Input: part model. Units: mm. Frame: model coordinates. Face numbers are marked on the shaded views. A direction names the side the tool comes from. Give positions to 0.01 mm unless a question says otherwise; leave off trailing zeros. Write each loop counter-clockwise with the first axis right and the second up, starting at its lowest first coordinate (ties: lowest second). Pieces come first, ordered by that corner, then holes. Notation, with made-up numbers: (-17, 36.5) - (12, 36.5) arc R30 cw to (12, 71.5) - close; hole circle Ø9 at (36.25, 26.25). An arc over 180 degrees is marked (long way). Answer as CSV lines item,"result".
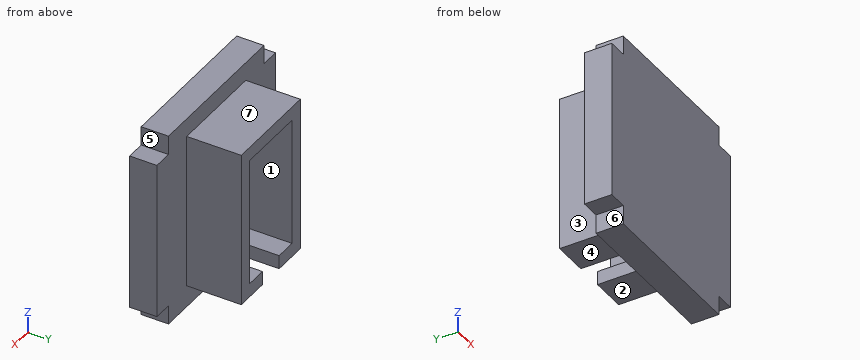
```python
from build123d import *

# Parameters (mm, degrees)
BOSS_EXTRUDE18_DEPTH = 5
BOSS_EXTRUDE19_DEPTH = 10


with BuildPart() as part:
    # Sketch21 → Boss-Extrude18 (new body)
    with BuildSketch(Plane(origin=(0, 0, 0), x_dir=(1, 0, 0), z_dir=(0, 1, 0))):
        Polygon((0, 17.98), (-14.48, 17.98), (-14.48, 14.48), (-17.98, 14.48), (-17.98, 0), (-17.98, -14.48), (-14.48, -14.48), (-14.48, -17.98), (0, -17.98), (14.48, -17.98), (14.48, -14.48), (17.98, -14.48), (17.98, 0), (17.98, 14.48), (14.48, 14.48), (14.48, 17.98), align=None)
    extrude(amount=BOSS_EXTRUDE18_DEPTH)

    # Sketch23 → Boss-Extrude19 (add)
    with BuildSketch(Plane(origin=(0, 5, 0), x_dir=(1, 0, 0), z_dir=(0, 1, 0))):
        Polygon((-8.95, 13.98), (-2.53, 13.98), (-2.53, 11.48), (-6.45, 11.48), (-6.45, -12.12), (6.45, -12.12), (6.45, 11.48), (2.53, 11.48), (2.53, 13.98), (8.95, 13.98), (8.95, -14.62), (-8.95, -14.62), align=None)
    extrude(amount=BOSS_EXTRUDE19_DEPTH)


solid = part.part
```
Item 1: Cut plane A-A on y = 2.75. Return the cut outline in (x, z), plus the area to 3 significant figures.
The answers:
outline,"(-17.98, -14.48) - (-14.48, -14.48) - (-14.48, -17.98) - (14.48, -17.98) - (14.48, -14.48) - (17.98, -14.48) - (17.98, 14.48) - (14.48, 14.48) - (14.48, 17.98) - (-14.48, 17.98) - (-14.48, 14.48) - (-17.98, 14.48) - close"
area,"1,240 mm²"
Item 2: Cut plane B-B on z = 0. Return the cut outline in (x, y).
The answers:
outline,"(-17.98, 0) - (17.98, 0) - (17.98, 5) - (8.95, 5) - (8.95, 15) - (6.45, 15) - (6.45, 5) - (-6.45, 5) - (-6.45, 15) - (-8.95, 15) - (-8.95, 5) - (-17.98, 5) - close"
Item 3: Ray query, line 1 (X direction, y = 6, z = -8); line 2 (Z direction, x = 5.5, y = 10.5); line 3 (Z direction, x = 2, y = 8). Return the intervals inside material, ascending. Write a range as from..to.
The answers:
line 1,"-8.95..-6.45, 6.45..8.95"
line 2,"-13.98..-11.48, 12.12..14.62"
line 3,"12.12..14.62"
Item 4: Cut plane C-C on x = 0. Return the cut outline in (y, z).
The answers:
outline,"(0, -17.98) - (5, -17.98) - (5, 12.12) - (15, 12.12) - (15, 14.62) - (5, 14.62) - (5, 17.98) - (0, 17.98) - close"
Item 5: Reachability of the marked faces 4, 5, 6 and 7 from +Z, -Z, +X, -X, +Y, -Y: full face, straight path, thin tool, end or side. Return the list, or none.
The answers:
face 4,"-Z, +X, -X, +Y"
face 5,"+Z, +X, +Y, -Y"
face 6,"-Z, -X, +Y, -Y"
face 7,"+Z, +X, -X, +Y"
Item 6: Contact query for flat-ended pins moving along their axis: pin 1 (5 mm diameter, centred on y = 12, z = -9, fed in from -X); pin 2 (1 mm diameter, centred on x = -16.5, y = 3.5, fed in from -Z); pin 3 (5 mm diameter, centred on x = -6.5, y = 6.5, fed in from +Z); pin 4 (2 mm diameter, centred on x = -4.5, y = 11.5, fed in from +Z). Output: stop coordinate, or through.
The answers:
pin 1,"x = -8.95"
pin 2,"z = -14.48"
pin 3,"z = 17.98"
pin 4,"z = 14.62"
Item 7: Mould query, pull axis X, two halves, no side actions, for the marked faces 1, 2 and 3. Classes: +X half, -X half, draft (parallel to the pull), parting line (faces both ways), or undercut.
The answers:
face 1,"undercut"
face 2,"draft"
face 3,"-X half"
Item 8: Cut plane D-D on x = 13.5. Return the cut outline in (y, z), plus the area to 3 significant figures.
The answers:
outline,"(0, -17.98) - (5, -17.98) - (5, 17.98) - (0, 17.98) - close"
area,"180 mm²"
